```python
from build123d import *

# Parameters (mm, degrees)
EXTRUDE_1_DEPTH     = 12
SKETCH_2_R          = 17
CUT_EXTRUDE_1_DEPTH = 13
FILLET_1_R          = 50
SKETCH_6_R          = 2.1
CUT_EXTRUDE_5_DEPTH = 13
SKETCH_8_R          = 23
CUT_EXTRUDE_6_DEPTH = 13
CUT_EXTRUDE_7_DEPTH = 13
SKETCH_12_W         = 2.62725081
SKETCH_12_H         = 4.213047789
EXTRUDE_4_DEPTH     = 2
SKETCH_13_R         = 2.56677592
EXTRUDE_5_DEPTH     = 2


with BuildPart() as part:
    # 草图1 → 凸台-拉伸1 (new body)
    with BuildSketch(Plane.XY):
        with BuildLine():
            Line((0.926524708, 29.985689119), (243.190486763, 22.5))
            ThreePointArc((243.190486763, 22.5), (305, 0), (243.190486763, -22.5))
            Line((243.190486763, -22.5), (0.926524708, -29.985689119))
            ThreePointArc((0.926524708, -29.985689119), (-30, 0), (0.926524708, 29.985689119))
        make_face()
    extrude(amount=EXTRUDE_1_DEPTH)

    # 草图2 → 切除-拉伸1 (cut, through all)
    with BuildSketch(Plane.XY.offset(12)):
        Circle(SKETCH_2_R)
    extrude(amount=-CUT_EXTRUDE_1_DEPTH, mode=Mode.SUBTRACT)

    # 圆角1
    fillet_1_edges = [part.edges().sort_by_distance(p)[0] for p in [
        (243.190486763, 22.5, 6),
        (243.190486763, -22.5, 6),
    ]]
    fillet(fillet_1_edges, radius=FILLET_1_R)

    # 草图6 → 切除-拉伸5 (cut, through all)
    with BuildSketch(Plane(origin=(0, 0, 0), x_dir=(-1, 0, 0), z_dir=(0, 0, -1))):
        with Locations((-242.5, 0)):
            Circle(SKETCH_6_R)
        with Locations((-248.933777814, -17.676659266)):
            Circle(SKETCH_6_R)
        with Locations((-265.224675114, -27.082213208)):
            Circle(SKETCH_6_R)
        with Locations((-283.75, -23.815698604)):
            Circle(SKETCH_6_R)
        with Locations((-295.841547072, -9.405553941)):
            Circle(SKETCH_6_R)
        with Locations((-295.841547072, 9.405553941)):
            Circle(SKETCH_6_R)
        with Locations((-283.75, 23.815698604)):
            Circle(SKETCH_6_R)
        with Locations((-265.224675114, 27.082213208)):
            Circle(SKETCH_6_R)
        with Locations((-248.933777814, 17.676659266)):
            Circle(SKETCH_6_R)
    extrude(amount=-CUT_EXTRUDE_5_DEPTH, mode=Mode.SUBTRACT)

    # 草图8 → 切除-拉伸6 (cut, through all)
    with BuildSketch(Plane(origin=(0, 0, 0), x_dir=(-1, 0, 0), z_dir=(0, 0, -1))):
        with Locations((-270, 0)):
            Circle(SKETCH_8_R)
    extrude(amount=-CUT_EXTRUDE_6_DEPTH, mode=Mode.SUBTRACT)

    # 草图9 → 切除-拉伸7 (cut, through all)
    with BuildSketch(Plane.XY.offset(12)):
        with BuildLine():
            Line((138.177203146, 7.265958797), (215.280000441, -10.340469156))
            ThreePointArc((215.280000441, -10.340469156), (222.197122435, -8.67472562), (225.051756781, -2.157644912))
            ThreePointArc((225.051756781, -2.157644912), (225.019683108, 1.330823929), (225.25794544, 4.811294392))
            ThreePointArc((225.25794544, 4.811294392), (223.604832456, 10.595836396), (218.388318749, 13.592783755))
            ThreePointArc((218.388318749, 13.592783755), (217.739691011, 13.685144373), (217.09211046, 13.784582076))
            Line((217.09211046, 13.784582076), (138.82229573, 13.190588508))
            ThreePointArc((138.82229573, 13.190588508), (135.862688972, 10.515405209), (138.177203146, 7.265958797))
        make_face()
        with BuildLine():
            Line((32.937456826, 12.295827459), (52.445209699, 12.46606904))
            ThreePointArc((52.445209699, 12.46606904), (55.323007544, 10.397995174), (54.221641474, 7.029665807))
            Line((54.221641474, 7.029665807), (36.230602759, -5.894048054))
            ThreePointArc((36.230602759, -5.894048054), (31.93419641, -6.130708054), (29.909058708, -2.334139502))
            ThreePointArc((29.909058708, -2.334139502), (29.893460188, 2.526071657), (29.093261442, 7.319982148))
            ThreePointArc((29.093261442, 7.319982148), (29.806984137, 10.741460671), (32.937456826, 12.295827459))
        make_face()
        with BuildLine():
            Line((51.481125102, -12.457655601), (86.617092144, -12.76428254))
            ThreePointArc((86.617092144, -12.76428254), (90.265824875, -10.479152721), (89.728149821, -6.207622039))
            Line((89.728149821, -6.207622039), (77.62420084, 8.354875892))
            ThreePointArc((77.62420084, 8.354875892), (73.771130602, 10.471180848), (69.509469202, 9.392691606))
            Line((69.509469202, 9.392691606), (49.182361686, -5.209117958))
            ThreePointArc((49.182361686, -5.209117958), (47.703176381, -9.666996809), (51.481125102, -12.457655601))
        make_face()
        with BuildLine():
            Line((103.223250725, -11.492707953), (90.577517941, 3.721620677))
            ThreePointArc((90.577517941, 3.721620677), (90.240211818, 8.363692898), (94.524430804, 10.18250504))
            Line((94.524430804, 10.18250504), (174.23015633, -7.595003002))
            ThreePointArc((174.23015633, -7.595003002), (176.557582723, -10.864575787), (173.550905727, -13.522942438))
            Line((173.550905727, -13.522942438), (106.264496118, -12.935742837))
            ThreePointArc((106.264496118, -12.935742837), (104.584684386, -12.549721733), (103.223250725, -11.492707953))
        make_face()
    extrude(amount=-CUT_EXTRUDE_7_DEPTH, mode=Mode.SUBTRACT)


with BuildPart() as body_2:
    # 草图12 → 凸台-拉伸4 (new body)
    with BuildSketch(Plane(origin=(0, 0, 0), x_dir=(0, 0, -1), z_dir=(1, 0, 0))):
        with Locations((1.313625405, 2.106523894)):
            Rectangle(SKETCH_12_W, SKETCH_12_H)
    extrude(amount=EXTRUDE_4_DEPTH)


with BuildPart() as body_3:
    # 草图13 → 凸台-拉伸5 (new body)
    with BuildSketch(Plane(origin=(0, 0, 0), x_dir=(0, 0, -1), z_dir=(1, 0, 0))):
        with Locations((-9.79748635, 0)):
            Circle(SKETCH_13_R)
    extrude(amount=EXTRUDE_5_DEPTH)


solid = part.part
```
The listing builds one solid part. Answer for the finished solid, in the listing's coordinates (mm). Coordinates: 2 decimals unless noted, no trailing zeros. Loops run counter-clockwise (first coordinate to the right, second up) from the corner with the lowest first, then second, coordinate; pieces in that order, holes last. Notation, with made-up numbers: (32.5, -15.5) - (46.5, -15.5) arc R30 cw to (46.5, 16.5) - close; hole circle Ø3 at (5.5, -35.75). An arc over 180 degrees is marked (long way). Use a Markdown table: item, result. Add a question column.
1) Given pin 1 (4 mm diameter, centred on y = 15.5, z = 3, fed in from +X); pin 2 (3 mm diameter, centred on y = 4.5, z = 4.5, fed in from -X); pin 3 (2 mm diameter, centred on x = 210, z = 6.5, fed in from -Y), each flat-ended and moving along its own axis, determine where each tip first touches the part or whether it passes through.
2) Find the intervals of material crossed by line 1 (Y direction, x = 147.5, z = 9.25); line 2 (Y direction, x = 283.75, z = 3.5); line 3 (Y direction, x = 174, z = 6), in increasing order.
3) The part is cut by section A-A, the plane x = -9. Give the vertices of the cut face in (y, z).
4) The part is cut by section B-B, the plane x = 167.5. Give the vertices of the cut face in (y, z), and give its area (3 significant figures).
5) The mould has two halves that part along Y. Classify faces 1 (the cylindrical face through (239.23, -24.68, 6.08)), 2 (the cylindrical face through (9.139, 14.334, 6.084)), 3 (the flat face through (139.8, 0.5, 12)), 4 (the cylindrical face through (47.683, -9.6, 6.084)): released by +Y, released by -Y, zero draft, split by the parting line, or undercut.
6) The part is cut by section C-C, the plane z = 9. State how many separate pieces and enclosed holes the cut face has, and give its area (3 significant figures).
Here are the results:
| question | item | result |
|---|---|---|
| 1 | pin 1 | stops at x = 302.29 |
| 1 | pin 2 | stops at x = -29.85 |
| 1 | pin 3 | stops at y = -23.56 |
| 2 | line 1 | y = -25.46 to -13.3, -1.63 to 5.14, 13.26 to 25.46 |
| 2 | line 2 | y = -32.19 to -25.92, -21.72 to -18.44, 18.44 to 21.72, 25.92 to 32.19 |
| 2 | line 3 | y = -24.64 to -13.49, -7.54 to -0.91, 13.46 to 24.64 |
| 3 | outline | (-28.62, 0) - (-14.42, 0) - (-14.42, 12) - (-28.62, 12) - close; (14.42, 0) - (28.62, 0) - (28.62, 12) - (14.42, 12) - close |
| 4 | outline | (-24.84, 0) - (-13.47, 0) - (-13.47, 12) - (-24.84, 12) - close; (-6.09, 0) - (0.57, 0) - (0.57, 12) - (-6.09, 12) - close; (13.41, 0) - (24.84, 0) - (24.84, 12) - (13.41, 12) - close |
| 4 | area | 354 mm^2 |
| 5 | face 1 | released by -Y |
| 5 | face 2 | undercut |
| 5 | face 3 | zero draft |
| 5 | face 4 | undercut |
| 6 | separate pieces | 1 |
| 6 | enclosed holes | 15 |
| 6 | area | 11,600 mm^2 |
